Part model, mm, in its own coordinate system. Coordinates: 2 decimals unless noted, no trailing zeros. Loops run counter-clockwise (first coordinate to the right, second up) from the corner with the lowest first, then second, coordinate; pieces in that order, holes last. Notation, with made-up numbers: (47, -34.5) - (84, -34.5) arc R9 cw to (84, -27.5) - close; hole circle Ø2 at (-23.5, -27.5). An arc over 180 degrees is marked (long way). Use a Markdown table: item, result. Add a question column.
1. Wall check: probe 1 along X at (y, z) = (5.25, 12.5); probe 2 along Y at (x, z) = (11, -18); probe 3 along Z at (x, y) = (57.5, 0.5). Give the ranges that are in metal, low to high. Write a range as [from, to].
2. Band-saw the part on B-B, the plane z = -12.5. Give the cut face in (x, y).
3. Band-saw the part on C-C, the plane x = 32.45. Give the cut face in (y, z), plus the area to 3 significant figures.
4. Band-saw the part on D-D, the plane x = -27. Give the cut face in (y, z), plus the area to 3 significant figures.
5. Drop flat-ended pins along their axis: pin 1 (4 mm diameter, centred on x = 19.5, y = 1, fed in from +Z); pin 2 (1.4 mm diameter, centred on x = -0.5, z = 12, fed in from -Y); pin 3 (5 mm diameter, centred on x = 0.5, z = -13, fed in from -Y). Give the stop position or say it passes through.
6. Band-saw the part on A-A, the plane y = 4. Give the cut face in (x, z).
from build123d import *

# Parameters (mm, degrees)
SKETCH1_W           = 129.8
SKETCH1_H           = 50
BOSS_EXTRUDE1_DEPTH = 9
SKETCH2_R           = 2.35
CUT_EXTRUDE1_DEPTH  = 8
CHAMFER1_SIZE       = 1
CHAMFER2_SIZE       = 10


with BuildPart() as part:
    # Sketch1 → Boss-Extrude1 (new body)
    with BuildSketch(Plane(origin=(0, 0, 0), x_dir=(1, 0, 0), z_dir=(0, 1, 0))):
        Rectangle(SKETCH1_W, SKETCH1_H)
    extrude(amount=BOSS_EXTRUDE1_DEPTH)

    # Sketch2 → Cut-Extrude1 (cut)
    with BuildSketch(Plane.XZ):
        with Locations(Location((-32.45, 12.5, 0), (0, 0, 270))):
            Circle(SKETCH2_R)
        with Locations(Location((0, 12.5, 0), (0, 0, 270))):
            Circle(SKETCH2_R)
        with Locations(Location((32.45, 12.5, 0), (0, 0, 270))):
            Circle(SKETCH2_R)
        with Locations(Location((32.45, -12.5, 0), (0, 0, 90))):
            Circle(SKETCH2_R)
        with Locations(Location((0, -12.5, 0), (0, 0, 90))):
            Circle(SKETCH2_R)
        with Locations(Location((-32.45, -12.5, 0), (0, 0, 90))):
            Circle(SKETCH2_R)
    extrude(amount=-CUT_EXTRUDE1_DEPTH, mode=Mode.SUBTRACT)

    # Chamfer1
    chamfer1_edges = [part.edges().sort_by_distance(p)[0] for p in [
        (-32.45, 0, -14.85),
        (0, 0, -14.85),
        (32.45, 0, -14.85),
        (32.45, 0, 14.85),
        (0, 0, 14.85),
        (-32.45, 0, 14.85),
    ]]
    chamfer(chamfer1_edges, length=CHAMFER1_SIZE)

    # Chamfer2
    # the kernel refuses this chamfer: 10 mm, written as the material it takes off along each edge
    with BuildSketch(Plane(origin=(90.61682988, 9, 25), x_dir=(0, -0.9996219169112968, 0.027495876610586317), z_dir=(-1, 0, 0)), Plane(origin=(-90.61682988, 9, -25), x_dir=(0, -0.9996219169112968, -0.027495876610586317), z_dir=(1, 0, 0))) as chamfer2_piece_1:
        Polygon((CHAMFER2_SIZE * 0.999621916911, -CHAMFER2_SIZE * 0.0274958766106), (-CHAMFER2_SIZE * 0.0274958766106, -CHAMFER2_SIZE * 0.999621916911), (0, 0), align=None)
    extrude(amount=181.233659759, mode=Mode.SUBTRACT)


solid = part.part
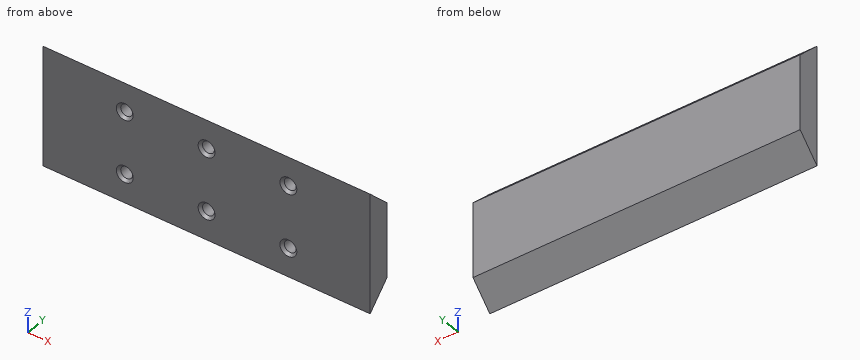
Geometry check:
| question | item | result |
|---|---|---|
| 1 | probe 1 | x = [-64.9, -34.8], [-30.1, -2.35], [2.35, 30.1], [34.8, 64.9] |
| 1 | probe 2 | y = [0, 6] |
| 1 | probe 3 | z = [-23.5, 23.5] |
| 2 | outline | (-64.9, 0) - (-35.8, 0) - (-34.8, 1) - (-34.8, 8) - (-30.1, 8) - (-30.1, 1) - (-29.1, 0) - (-3.35, 0) - (-2.35, 1) - (-2.35, 8) - (2.35, 8) - (2.35, 1) - (3.35, 0) - (29.1, 0) - (30.1, 1) - (30.1, 8) - (34.8, 8) - (34.8, 1) - (35.8, 0) - (64.9, 0) - (64.9, 9) - (-64.9, 9) - close |
| 3 | outline | (0, -24) - (9, -15) - (9, 15) - (0, 24) - (0, 15.85) - (1, 14.85) - (8, 14.85) - (8, 10.15) - (1, 10.15) - (0, 9.15) - (0, -9.15) - (1, -10.15) - (8, -10.15) - (8, -14.85) - (1, -14.85) - (0, -15.85) - close |
| 3 | area | 274 mm^2 |
| 4 | outline | (0, -24) - (9, -15) - (9, 15) - (0, 24) - close |
| 4 | area | 351 mm^2 |
| 5 | pin 1 | stops at z = 24 |
| 5 | pin 2 | stops at y = 8 |
| 5 | pin 3 | stops at y = 0.14 |
| 6 | outline | (-64.9, -20) - (64.9, -20) - (64.9, 20) - (-64.9, 20) - close; hole circle Ø4.7 at (-32.45, -12.5); hole circle Ø4.7 at (-32.45, 12.5); hole circle Ø4.7 at (0, -12.5); hole circle Ø4.7 at (0, 12.5); hole circle Ø4.7 at (32.45, -12.5); hole circle Ø4.7 at (32.45, 12.5) |
